```python
from build123d import *

# Parameters (mm, degrees)
SKETCH1_W               = 466
SKETCH1_H               = 500
BOSS_EXTRUDE1_DEPTH     = 2
SKETCH2_W               = 2
SKETCH2_H               = 40
BOSS_EXTRUDE2_DEPTH     = 40
FILLET1_R               = 10
SKETCH3_R               = 4
CUT_EXTRUDE1_DEPTH      = 531.490339215
CROQUIS2_W              = 40
CROQUIS2_H              = 40
CORTAR_EXTRUIR1_DEPTH   = 10
CROQUIS3_W              = 40
CROQUIS3_H              = 40
CORTAR_EXTRUIR2_DEPTH   = 10
CROQUIS4_W              = 2
CROQUIS4_H              = 40
SALIENTE_EXTRUIR1_DEPTH = 40
CROQUIS5_R              = 4
CORTAR_EXTRUIR3_DEPTH   = 516.620984833
REDONDEO1_R             = 10


with BuildPart() as part:
    # Sketch1 → Boss-Extrude1 (new body)
    with BuildSketch(Plane(origin=(0, 0, 0), x_dir=(1, 0, 0), z_dir=(0, 1, 0))):
        Rectangle(SKETCH1_W, SKETCH1_H)
    extrude(amount=BOSS_EXTRUDE1_DEPTH)

    # Sketch2 → Boss-Extrude2 (add)
    with BuildSketch(Plane(origin=(0, 2, 0), x_dir=(1, 0, 0), z_dir=(0, 1, 0))):
        with Locations((232, -230)):
            Rectangle(SKETCH2_W, SKETCH2_H)
        with Locations((232, 230)):
            Rectangle(SKETCH2_W, SKETCH2_H)
        with Locations((-232, 230)):
            Rectangle(SKETCH2_W, SKETCH2_H)
        with Locations((-232, -230)):
            Rectangle(SKETCH2_W, SKETCH2_H)
        with Locations((215, -230)):
            Rectangle(SKETCH2_W, SKETCH2_H)
        with Locations((-215, -230)):
            Rectangle(SKETCH2_W, SKETCH2_H)
        with Locations((-215, 230)):
            Rectangle(SKETCH2_W, SKETCH2_H)
        with Locations((215, 230)):
            Rectangle(SKETCH2_W, SKETCH2_H)
    extrude(amount=BOSS_EXTRUDE2_DEPTH)

    # Fillet1
    fillet1_edges = [part.edges().sort_by_distance(p)[0] for p in [
        (232, 42, 210),
        (232, 42, 250),
        (232, 42, -250),
        (232, 42, -210),
        (-232, 42, -250),
        (-232, 42, -210),
        (-232, 42, 250),
        (-232, 42, 210),
        (-215, 42, 250),
        (-215, 42, 210),
        (215, 42, 210),
        (215, 42, 250),
        (-215, 42, -210),
        (-215, 42, -250),
        (215, 42, -210),
        (215, 42, -250),
    ]]
    fillet(fillet1_edges, radius=FILLET1_R)

    # Sketch3 → Cut-Extrude1 (cut, through all)
    with BuildSketch(Plane.ZY.offset(233)):
        with Locations((-230, 22)):
            Circle(SKETCH3_R)
        with Locations((230, 22)):
            Circle(SKETCH3_R)
    extrude(amount=-CUT_EXTRUDE1_DEPTH, mode=Mode.SUBTRACT)

    # Croquis2 → Cortar-Extruir1 (cut)
    with BuildSketch(Plane.ZY.offset(233)):
        with Locations((230, 22)):
            Rectangle(CROQUIS2_W, CROQUIS2_H)
    extrude(amount=-CORTAR_EXTRUIR1_DEPTH, mode=Mode.SUBTRACT)

    # Croquis3 → Cortar-Extruir2 (cut)
    with BuildSketch(Plane(origin=(233, 0, 0), x_dir=(0, 0, -1), z_dir=(1, 0, 0))):
        with Locations((-230, 22)):
            Rectangle(CROQUIS3_W, CROQUIS3_H)
    extrude(amount=-CORTAR_EXTRUIR2_DEPTH, mode=Mode.SUBTRACT)

    # Croquis4 → Saliente-Extruir1 (add)
    with BuildSketch(Plane(origin=(0, 2, 0), x_dir=(1, 0, 0), z_dir=(0, 1, 0))):
        with Locations((-198, -230)):
            Rectangle(CROQUIS4_W, CROQUIS4_H)
        with Locations((198, -230)):
            Rectangle(CROQUIS4_W, CROQUIS4_H)
    extrude(amount=SALIENTE_EXTRUIR1_DEPTH)

    # Croquis5 → Cortar-Extruir3 (cut, through all)
    with BuildSketch(Plane.ZY.offset(216)):
        with Locations((230, 22)):
            Circle(CROQUIS5_R)
    extrude(amount=-CORTAR_EXTRUIR3_DEPTH, mode=Mode.SUBTRACT)

    # Redondeo1
    redondeo1_edges = [part.edges().sort_by_distance(p)[0] for p in [
        (-198, 42, 250),
        (-198, 42, 210),
        (198, 42, 210),
        (198, 42, 250),
    ]]
    fillet(redondeo1_edges, radius=REDONDEO1_R)


solid = part.part
```
Here's how the part is built. I have some questions about the finished solid (model axes, mm). A direction names the side the tool comes from. Give positions to 0.01 mm unless a question says otherwise; leave off trailing zeros. Loops run counter-clockwise (first coordinate to the right, second up) from the corner with the lowest first, then second, coordinate; pieces in that order, holes last. Notation, with made-up numbers: M 63.25,78 L 78.25,78 A23 ccw 78.25,105 Z; hole C 36,-26 d8. An arc over 180 degrees is marked long. Use one line per item in the form item = value. Start each with the question number.
Q1. Thinking about a two-plate mould opening in X: for faces 3 (the flat face through (216, 17, 230)), 4 (the flat face through (216, 17, -230)), 5 (the flat face through (-216, 17, 230)), which applies, +X half, -X half, draft (parallel to the pull), parting line (faces both ways), or undercut?
Q2. Which directions (+Z, -Z, +X, -X, +Y, -Y) give clear straight access to the entire face, cutting with the end or side of a thin tool? Please do faces 1 (the flat face through (214, 17, 230)), 2 (the flat face through (-233, 1, -147)).
Q3. If we section it at C-C (z = -23): Write out the boundary of the cut face in (x, y).
Q4. Will these pins go through, and if not, where does the flat tip stop? pin 1 Ø7 at (y, z) = (22, -230) entering from +X; pin 2 Ø13 at (y, z) = (22, 230) entering from +X; pin 3 Ø20 at (y, z) = (31, 226.5) entering from -X; pin 4 Ø1.6 at (x, y) = (-197.5, 20) entering from -Z.
Q5. I need wall thicknesses on line 1 along Y through (x, z) = (-215.55, 230); line 2 along X through (y, z) = (26, 221); line 3 along Y through (x, z) = (-35, 138.5). Which ranges of each line are inside material? Lowest first, please.
Q6. If we section it at A-A (y = 11.5): State how many separate pieces and enclosed holes the cut face has, then the cut area to 3 significant figures.
Q7. If we section it at B-B (x = -143): Write out the boundary of the cut face in (y, z), then the cut area to 3 significant figures.
Taken from the geometry:
q1.face_3 = +X half
q1.face_4 = undercut
q1.face_5 = -X half
q2.face_1 = +Z, -Z, +Y
q2.face_2 = +Z, -Z, -X, +Y, -Y
q3.outline = M -233,0 L 233,0 L 233,2 L -233,2 Z
q4.pin_1 = through
q4.pin_2 = 216
q4.pin_3 = -216
q4.pin_4 = 210
q5.line_1 = 0 to 18, 26 to 42
q5.line_2 = -216 to -214, -199 to -197, 197 to 199, 214 to 216
q5.line_3 = 0 to 2
q6.separate_pieces = 8
q6.enclosed_holes = 0
q6.area = 640 mm^2
q7.outline = M 0,-250 L 2,-250 L 2,250 L 0,250 Z
q7.area = 1,000 mm^2
